```python
from build123d import *

# Parameters (mm, degrees)
EXTRUDE_1_DEPTH          = 10
CUT_EXTRUDE_1_DEPTH      = 16
CUT_EXTRUDE_1_DEPTH_BACK = 16
SKETCH_2_R               = 1.6
SKETCH_2_W               = 6.5
SKETCH_2_H               = 10
FILLET_1_R               = 1.5


with BuildPart() as part:
    # 草图1 → 凸台-拉伸1 (new, symmetric)
    with BuildSketch(Plane.XY):
        with BuildLine():
            Line((0, -3.25), (-10, -3.25))
            Line((-10, -3.25), (-10, -1.75))
            Line((-10, -1.75), (-2.738612788, -1.75))
            ThreePointArc((-2.738612788, -1.75), (1.5612495, 2.850438563), (0, -3.25))
        make_face()
    extrude(amount=EXTRUDE_1_DEPTH, both=True)

    # 草图2 → 切除-拉伸1 (cut, two sides: drawn at the far end of the back side and taken through both)
    with BuildSketch(Plane(origin=(0, -1.75, 0), x_dir=(1, 0, 0), z_dir=(0, 1, 0)).offset(-CUT_EXTRUDE_1_DEPTH_BACK)):
        with Locations(Location((-7, -6, 0), (0, 0, 270))):
            Circle(SKETCH_2_R)
        with Locations(Location((-7, 6, 0), (0, 0, 90))):
            Circle(SKETCH_2_R)
        Rectangle(SKETCH_2_W, SKETCH_2_H)
    extrude(amount=CUT_EXTRUDE_1_DEPTH + CUT_EXTRUDE_1_DEPTH_BACK, mode=Mode.SUBTRACT)

    # 圆角1
    fillet_1_edges = [part.edges().sort_by_distance(p)[0] for p in [
        (-10, -2.5, 10),
        (-10, -2.5, -10),
    ]]
    fillet(fillet_1_edges, radius=FILLET_1_R)


solid = part.part
```
Verification items for the finished model (mm, model axes). A direction names the side the tool comes from. Round coordinates to 2 decimals unless told otherwise and drop trailing zeros. Order: outer loops, then holes, each group sorted by start corner. A loop starts at its lowest first (then second) coordinate and runs counter-clockwise, first axis right, second up. Notation, with made-up numbers: (73.5, 77) -> (89.5, 77) arc R26 cw to (89.5, 104) -> close; hole circle Ø1 at (-6.75, -39). An arc over 180 degrees is marked (long way). Put each result on its own line as item: value. Start each with the question number.
(1) Section check D-D (y = -2.25). Enter the section's corners in (x, z), then the cut area to 3 significant figures.
(2) Section check C-C (z = -6). Enter the section's corners in (x, y), then the cut area to 3 significant figures.
(3) Draft check along X on faces 1 (the face through (-6, -3.25, 0)), 2 (the face through (-9.57, -2.49, 9.55)), 3 (the face through (-8.42, -2.51, 6.74)). Enter one of: +X half, -X half, draft (parallel to the pull), parting line (faces both ways), or undercut.
(4) Material ranges on line 1 along Z through (x, y) = (-2.75, -1.5); line 2 along Y through (x, z) = (-9, -6.25); line 3 along X through (y, z) = (-2.5, 6), recorded low to high.
(5) Section check A-A (x = -7). Enter the section's corners in (y, z), then the cut area to 3 significant figures.
(6) Section check B-B (y = -1.25). Enter the section's corners in (x, z).
(7) Tool access check on faces 4 (the face through (-1, -1, 10)), 5 (the face through (0, 0, -5)). Record the directions out of +Z, -Z, +X, -X, +Y, -Y that give a thin tool (end or side, any length) a straight path to the whole face; none if there is none.
(8) Depth check by flat-ended pin: pin 1 Ø1.5 at (x, z) = (0.5, -3) entering from +Y; pin 2 Ø1.6 at (y, z) = (-2.5, 0) entering from +X; pin 3 Ø3.5 at (x, z) = (-6.5, -3) entering from +Y. Enter the tip coordinate at first touch or a pass-through.
Completed:
1. outline: (-10, -8.5) arc R1.5 ccw to (-8.5, -10) -> (2.35, -10) -> (2.35, -5) -> (-3.25, -5) -> (-3.25, 5) -> (2.35, 5) -> (2.35, 10) -> (-8.5, 10) arc R1.5 ccw to (-10, 8.5) -> close; hole circle Ø3.2 at (-7, -6); hole circle Ø3.2 at (-7, 6)
1. area: 174 mm2
2. outline: (-10, -3.25) -> (-8.6, -3.25) -> (-8.6, -1.75) -> (-10, -1.75) -> close; (-5.4, -3.25) -> (0, -3.25) arc R3.25 ccw (long way) to (-2.74, -1.75) -> (-5.4, -1.75) -> close
2. area: 40.5 mm2
3. face 1: draft
3. face 2: -X half
3. face 3: undercut
4. line 1: z = -10 to -5, 5 to 10
4. line 2: y = -3.25 to -1.75
4. line 3: x = -10 to -8.6, -5.4 to 2.08
5. outline: (-3.25, -10) -> (-1.75, -10) -> (-1.75, -7.6) -> (-3.25, -7.6) -> close; (-3.25, -4.4) -> (-1.75, -4.4) -> (-1.75, 4.4) -> (-3.25, 4.4) -> close; (-3.25, 7.6) -> (-1.75, 7.6) -> (-1.75, 10) -> (-3.25, 10) -> close
5. area: 20.4 mm2
6. outline: (-3, -10) -> (3, -10) -> (3, -5) -> (-3, -5) -> close; (-3, 5) -> (3, 5) -> (3, 10) -> (-3, 10) -> close
7. face 4: +Z, +X, -X, +Y, -Y
7. face 5: +X, +Y, -Y
8. pin 1: passes through
8. pin 2: stops at x = -3.25
8. pin 3: stops at y = -1.75
